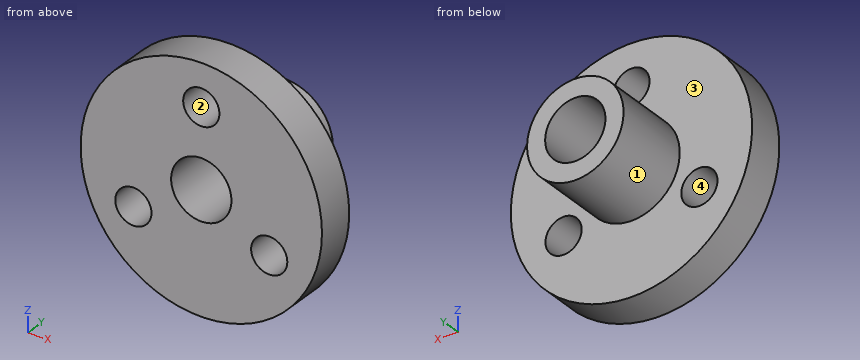
```python
from build123d import *

# Parameters (mm, degrees)
ESBO_O1_R                = 10
ESBO_O1_R_2              = 2.5
RESSALTO_EXTRUS_O1_DEPTH = 3.2
ESBO_O2_R                = 1.5
CORTE_EXTRUS_O1_DEPTH    = 3.2
PADR_OCIRCULAR1_COUNT    = 3
ESBO_O3_R                = 4
ESBO_O3_R_2              = 2.5
RESSALTO_EXTRUS_O2_DEPTH = 6.6


with BuildPart() as part:
    # Esboço1 → Ressalto-extrusão1 (new body)
    with BuildSketch(Plane(origin=(0, 0, 0), x_dir=(1, 0, 0), z_dir=(0, 1, 0))):
        Circle(ESBO_O1_R)
        Circle(ESBO_O1_R_2, mode=Mode.SUBTRACT)
    extrude(amount=RESSALTO_EXTRUS_O1_DEPTH)

    # Esboço2 → Corte-extrusão1 (cut)
    with BuildSketch(Plane.XZ):
        with Locations((0, 6.5)):
            Circle(ESBO_O2_R)
    corte_extrus_o1 = extrude(amount=-CORTE_EXTRUS_O1_DEPTH, mode=Mode.SUBTRACT)

    # PadrãoCircular1: Corte-extrusão1 ×3 about axis
    padr_ocircular1_axis = Axis((0, 0, 0), (0, 1, 0))
    for i in range(1, PADR_OCIRCULAR1_COUNT):
        add(corte_extrus_o1.rotate(padr_ocircular1_axis, i * 360 / PADR_OCIRCULAR1_COUNT), mode=Mode.SUBTRACT)

    # Esboço3 → Ressalto-extrusão2 (add)
    with BuildSketch(Plane(origin=(0, 3.2, 0), x_dir=(1, 0, 0), z_dir=(0, 1, 0))):
        Circle(ESBO_O3_R)
        Circle(ESBO_O3_R_2, mode=Mode.SUBTRACT)
    extrude(amount=RESSALTO_EXTRUS_O2_DEPTH)


solid = part.part
```
The listing builds one solid part. Answer for the finished solid, in the listing's coordinates (mm). Face numbers are marked on the shaded views. Give positions to 0.01 mm unless a question says otherwise; leave off trailing zeros. Order: outer loops, then holes, each group sorted by start corner. A loop starts at its lowest first (then second) coordinate and runs counter-clockwise, first axis right, second up. Notation, with made-up numbers: (62.5, 56.25) -> (100.5, 56.25) arc R10 cw to (100.5, 75.25) -> close; hole circle Ø8 at (16.25, 15). An arc over 180 degrees is marked (long way). Write each question's results on one line, items separated by ' | '.
Q1. The part is cut by section D-D, the plane z = -3.25. Give the vertices of the cut face in (x, y).
Checked values:
outline: (-9.46, 0) -> (-7.13, 0) -> (-7.13, 3.2) -> (-9.46, 3.2) -> close; (-4.13, 0) -> (4.13, 0) -> (4.13, 3.2) -> (2.33, 3.2) -> (2.33, 9.8) -> (-2.33, 9.8) -> (-2.33, 3.2) -> (-4.13, 3.2) -> close; (7.13, 0) -> (9.46, 0) -> (9.46, 3.2) -> (7.13, 3.2) -> close
Q2. Each of these flat-tipped pins is pushed along its axis until it touches: P1, Ø6, axis at x = 6.5, z = 6.5, coming from the -Y side; P2, Ø3, axis at x = 0, z = 0, coming from the +Y side; P3, Ø3.5, axis at x = 0, z = 6.5, coming from the +Y side; P4, Ø3, axis at x = 8, y = 2.5, coming from the -Z side. Where does it stop, or does it pass through?
Checked values:
P1: stops at y = 0 | P2: passes through | P3: stops at y = 3.2 | P4: stops at z = -7.6
Q3. The part is cut by section C-C, the plane x = 4.5. Give the vertices of the cut face in (y, z).
Checked values:
outline: (0, -8.93) -> (3.2, -8.93) -> (3.2, -4.24) -> (0, -4.24) -> close; (0, -2.26) -> (3.2, -2.26) -> (3.2, 8.93) -> (0, 8.93) -> close
Q4. The part is cut by section A-A, the plane x = 0. Give the vertices of the cut face in (y, z), and give its area (3 significant figures).
Checked values:
outline: (0, -10) -> (3.2, -10) -> (3.2, -4) -> (9.8, -4) -> (9.8, -2.5) -> (0, -2.5) -> close; (0, 2.5) -> (9.8, 2.5) -> (9.8, 4) -> (3.2, 4) -> (3.2, 5) -> (0, 5) -> close; (0, 8) -> (3.2, 8) -> (3.2, 10) -> (0, 10) -> close | area: 58.2 mm^2
Q5. The part is cut by section B-B, the plane z = 6.5. Give the vertices of the cut face in (x, y), and give its area (3 significant figures).
Checked values:
outline: (-7.6, 0) -> (-1.5, 0) -> (-1.5, 3.2) -> (-7.6, 3.2) -> close; (1.5, 0) -> (7.6, 0) -> (7.6, 3.2) -> (1.5, 3.2) -> close | area: 39.0 mm^2
Q6. Determine the mould class of the marked faces 1, 2, 3 and 4 for opening direction X: pulls with the +X half, pulls with the -X half, needs draft (parallel to the pull), parting line crosses it, or undercut.
Checked values:
face 1: parting line crosses it | face 2: undercut | face 3: needs draft | face 4: undercut
Q7. Straight lines are drawn through the part: probe 1 along Z at (x, y) = (0, 0.75); probe 2 along Z at (x, y) = (-1.25, 1); probe 3 along Y at (x, z) = (-1.5, -6.75). For each, find the intervals that lie inside material, in ascending order. Write a range as from..to.
Checked values:
probe 1: z = -10..-2.5, 2.5..5, 8..10 | probe 2: z = -9.92..-2.17, 2.17..5.67, 7.33..9.92 | probe 3: y = 0..3.2
